Check sheet for the modelled part. Datum: model origin and axes. Units: mm. A direction names the side the tool comes from. Give positions to 0.01 mm unless a question says otherwise; leave off trailing zeros. Loops run counter-clockwise (first coordinate to the right, second up) from the corner with the lowest first, then second, coordinate; pieces in that order, holes last. Notation, with made-up numbers: M 49.25,58 L 65.25,58 A22 ccw 65.25,71 Z; hole C 30,24 d1. An arc over 180 degrees is marked long. Use one line per item in the form item = value.
Autodesk Inventor part; units mm, degrees
ref_plane "YZ Plane" through (0, 0, 0) normal (1, 0, 0) x (0, 1, 0)
ref_plane "XZ Plane" through (0, 0, 0) normal (0, 1, 0) x (-1, 0, 0)
ref_plane "XY Plane" through (0, 0, 0) normal (0, 0, 1) x (1, 0, 0)
sketch "Sketch1" plane through (0, 0, 0) normal (0, 0, 1) x (1, 0, 0)
  line L0 (-15, 7.5) -> (15, 7.5) construction
  line L1 (0, 11.0799) -> (0, -11.0799)
  line L2 (-15, 7.5) -> (-15, -7.5) construction
  line L3 (-15, 3.1) -> (-15, -3.1) construction
  line L4 (-15, 7.5) -> (-15, 3.1) construction
  line L5 (-15, 7.5) -> (-3.1, 7.5) construction
  line L6 (-15, 3.1) -> (-13, 3.1)
  line L7 (-3.1, 5.5) -> (-3.1, 7.5)
  line L8 (-13, 3.1) -> (-13, 5.5) construction
  line L9 (-15, 3.1) -> (-9, 3.1) construction
  line L10 (-13, 5.5) -> (-9, 3.1) construction
  line L11 (-9, 0) -> (-9, 3.1)
  line L12 (-21.4971, 0) -> (21.0828, 0)
  line L13 (-9, 0) -> (-9, -3.1) construction
  line L14 (-9, -3.1) -> (-13, -5.5) construction
  line L15 (-13, -5.5) -> (-13, -3.1) construction
  line L16 (-13, -3.1) -> (-15, -3.1)
  line L17 (-15, -3.1) -> (-15, -7.5) construction
  line L18 (-15, -7.5) -> (0, -7.5) construction
  line L19 (0, -7.5) -> (0, -5.5)
  line L20 (0, -5.5) -> (-9.1127, -5.5) construction
  line L21 (-9.1127, -5.5) -> (-7, -4.2324) construction
  line L22 (-7, -4.2324) -> (-7, 3.2725) construction
  line L23 (0, 0) -> (-3.1, 0)
  line L24 (-7, 3.2725) -> (-3.1, 0) construction
  line L25 (-3.1, 5.5) -> (-7, 5.5)
  line L26 (-7, 5.5) -> (-3.1, 1.9884)
  line L27 (-3.1, 1.9884) -> (0, 1.9884)
  line L28 (0, 1.9884) -> (0, 0)
  arc A0 (-13, 7.5) -> (-15, 5.5) centre (-13, 5.5) ccw
  line L29 (-13, 7.5) -> (-3.1, 7.5)
  line L30 (-15, 5.5) -> (-15, 3.1)
  arc A1 (-12.6971, 5.3183) -> (-13, 5.1468) centre (-12.8, 5.1468) ccw
  line L31 (-13, 5.1468) -> (-13, 3.1)
  line L32 (-12.6971, 5.3183) -> (-9, 3.1)
  arc A2 (-13, -5.1468) -> (-12.6971, -5.3183) centre (-12.8, -5.1468) ccw
  line L33 (-13, -5.1468) -> (-13, -3.1)
  line L34 (-12.6971, -5.3183) -> (-9, -3.1) construction
  arc A3 (-15, -5.5) -> (-13, -7.5) centre (-13, -5.5) ccw
  line L35 (-15, -5.5) -> (-15, -3.1)
  line L36 (-13, -7.5) -> (0, -7.5)
  arc A4 (-8.4935, -5.1285) -> (-8.3906, -5.5) centre (-8.3906, -5.3) ccw
  line L37 (-8.4935, -5.1285) -> (-7, -4.2324) construction
  line L38 (-8.3906, -5.5) -> (0, -5.5)
  arc A5 (-7.0971, -4.2906) -> (-7, -4.1191) centre (-7.2, -4.1191) ccw
  line L39 (-8.4935, -5.1285) -> (-7.0971, -4.2906)
  line L40 (-7, -4.1191) -> (-7, 3.2725) construction
  arc A6 (-9.0971, -3.1583) -> (-9, -2.9868) centre (-9.2, -2.9868) ccw
  line L41 (-9, -2.9868) -> (-9, 0)
  line L42 (-9.0971, -3.1583) -> (-12.6971, -5.3183)
  arc A7 (-6.6714, 2.9968) -> (-7, 2.8436) centre (-6.8, 2.8436) ccw
  line L43 (-7, -4.1191) -> (-7, 2.8436)
  line L44 (-3.1, 0) -> (-6.6714, 2.9968)
  line L45 (-3.1, 0) -> (0, 0)
  point P0 (0, 7.5)
  point P1 (-15, 0)
  dimension "d0" = 7.5
  dimension "d1" = 30
  dimension "d2" = 15
  dimension "d3" = 6.2
  dimension "d4" = 3.1
  dimension "d5" = 2
  dimension "d6" = 2.4
  dimension "d7" = 6
  dimension "d8" = 3.1
  dimension "d9" = 2
  dimension "d10" = 2
  dimension "d11" = 2
  dimension "d12" = 50
  dimension "d13" = 2
  dimension "outer_angle" = 2
  dimension "inner_angle" = 0.2
  dimension "d18" = 0.2
  dimension "d19" = 2
  dimension "d20" = 0.2
  dimension "d21" = 0.2
  dimension "d22" = 0.2
  dimension "d23" = 0.2
extrude "Extrusion2" add sketch "Sketch1" along normal mid plane 100 contours L1 L12 L44 A7 L43 L11 L32 A1 L31 L6 L30 A0 L29 L7 L25 L26 L27 | L1 L36 A3 L35 L16 L33 A2 L42 A6 L41 L12 L43 A5 L39 A4 L38
mirror "Mirror2" about plane through (0, 0, 0) normal (1, 0, 0) of "Extrusion2"
equation "\"d18\" = inner_angle"
equation "\"d19\" = outer_angle"
equation "\"d20\" = inner_angle"
equation "\"d21\" = inner_angle"
equation "\"d22\" = inner_angle"
equation "\"d23\" = inner_angle"
properties part number "profile_15x60"
1) Section check B-B (x = -11). Record the cut outline in (y, z).
Evaluation:
outline = M -7.5,-50 L -4.3,-50 L -4.3,50 L -7.5,50 Z; M 4.3,-50 L 7.5,-50 L 7.5,50 L 4.3,50 Z
2) Release check for a two-part mould opening along X. For faces 4 (the face through (15, -4, -1)), 5 (the face through (13, 4, -1)), 6 (the face through (4.91, 1.52, -0.7)), 7 (the face through (0, -7.5, -1)) record: pulls with the +X half, pulls with the -X half, needs draft (parallel to the pull), parting line crosses it, or undercut.
Evaluation:
face_4 = pulls with the +X half
face_5 = undercut
face_6 = undercut
face_7 = needs draft
3) Set-up check for faces 1 (the face through (-14, 3.1, -1)), 2 (the face through (14, 3.1, -1)), 3 (the face through (-7, -1, -1)): record each of +Z, -Z, +X, -X, +Y, -Y from which the full face is reachable in a straight line by a thin tool's end or side.
Evaluation:
face_1 = +Z, -Z, -X
face_2 = +Z, -Z, +X
face_3 = +Z, -Z
4) Section check A-A (y = -2). Record the cut outline in (x, z), then the cut area to 3 significant figures.
Evaluation:
outline = M -9,-50 L -7,-50 L -7,50 L -9,50 Z; M 7,-50 L 9,-50 L 9,50 L 7,50 Z
area = 400 mm^2
5) Scan lines: line 1 (Y direction, x = 2.5, z = 43); line 2 (X direction, y = 1.75, z = 38); line 3 (Y direction, x = -6.25, z = -36.5). Record each from-to range of solid material in increasing order.
Evaluation:
line_1 = -7.5 to -5.5, 0 to 1.99
line_2 = -9 to -7, -5.19 to 5.19, 7 to 9
line_3 = -7.5 to -5.5, 2.64 to 4.82, 5.5 to 7.5
6) Depth check by flat-ended pin: pin 1 Ø1 at (x, z) = (14, -19.5) entering from -Y; pin 2 Ø3 at (y, z) = (-1, -7) entering from -X; pin 3 Ø5 at (y, z) = (-2.5, -11) entering from -X; pin 4 Ø3 at (y, z) = (-1, -14) entering from +X. Enter the tip coordinate at first touch or a pass-through.
Evaluation:
pin_1 = -7.44
pin_2 = -9
pin_3 = -15
pin_4 = 9
7) Section check C-C (y = 4). Record the cut outline in (x, z), then the cut area to 3 significant figures.
Evaluation:
outline = M -15,-50 L -13,-50 L -13,50 L -15,50 Z; M -10.5,-50 L -5.33,-50 L -5.33,50 L -10.5,50 Z; M 5.33,-50 L 10.5,-50 L 10.5,50 L 5.33,50 Z; M 13,-50 L 15,-50 L 15,50 L 13,50 Z
area = 1,430 mm^2
